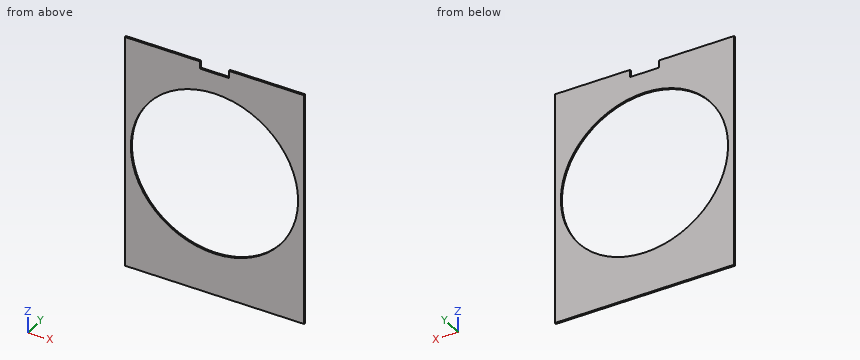
from build123d import *

# Parameters (mm, degrees)
SKETCH4_W           = 381
SKETCH4_H           = 508
BOSS_EXTRUDE1_DEPTH = 3.81
SKETCH5_R           = 177.8
CUT_EXTRUDE1_DEPTH  = 789.432041398
SKETCH6_W           = 62
SKETCH6_H           = 16
CUT_EXTRUDE2_DEPTH  = 789.432041398


with BuildPart() as part:
    # Sketch4 → Boss-Extrude1 (new body)
    with BuildSketch(Plane(origin=(190.463297595, 0, 436.273520924), x_dir=(1, 0, 0), z_dir=(0, 1, 0))):
        Rectangle(SKETCH4_W, SKETCH4_H)
    extrude(amount=BOSS_EXTRUDE1_DEPTH)

    # Sketch5 → Cut-Extrude1 (cut, through all)
    with BuildSketch(Plane(origin=(0, 3.81, 0), x_dir=(1, 0, 0), z_dir=(0, 1, 0))):
        with Locations(Location((190.463297595, -451.583397082, 0), (0, 0, 270))):
            Circle(SKETCH5_R)
    extrude(amount=-CUT_EXTRUDE1_DEPTH, mode=Mode.SUBTRACT)

    # Sketch6 → Cut-Extrude2 (cut, through all)
    with BuildSketch(Plane(origin=(0, 3.81, 0), x_dir=(1, 0, 0), z_dir=(0, 1, 0))):
        with Locations((190.463297595, -682.273520924)):
            Rectangle(SKETCH6_W, SKETCH6_H)
    extrude(amount=-CUT_EXTRUDE2_DEPTH, mode=Mode.SUBTRACT)


solid = part.part
Part model, mm, in its own coordinate system. Coordinates: 2 decimals unless noted, no trailing zeros. Loops run counter-clockwise (first coordinate to the right, second up) from the corner with the lowest first, then second, coordinate; pieces in that order, holes last. Notation, with made-up numbers: M -7.75,31.25 L 15.25,31.25 A25 cw 15.25,70.25 Z; hole C 58.25,-6 d8. An arc over 180 degrees is marked long. Use a Markdown table: item, result. Add a question column.
Q1. Cut at C-C (y = 1.85). Write the cut outline in (x, z), and give its area (3 significant figures).
Q2. Pin check, flat tip, straight feed: P1, Ø1.9, axis at x = 202.5, y = 1, coming from the +Z side. Stop position of the tip, or through.
Q3. Cut at B-B (z = 281.5). Write the cut outline in (x, y), and give its area (3 significant figures).
Q4. Probe L1, parallel to X at y = 0.55, z = 584; L2, parallel to X at y = 1.6, z = 519.5; L3, parallel to Z at x = 242, y = 2.3. List the from-to ranges inside material, lowest first.
Q5. Cut at A-A (x = 142). Write the cut outline in (y, z), and give its area (3 significant figures).
Worked out:
| question | item | result |
|---|---|---|
| 1 | outline | M -0.04,182.27 L 380.96,182.27 L 380.96,690.27 L 221.46,690.27 L 221.46,674.27 L 159.46,674.27 L 159.46,690.27 L -0.04,690.27 Z; hole C 190.46,451.58 d355.6 |
| 1 | area | 93,200 mm2 |
| 2 | P1 | stops at z = 674.27 |
| 3 | outline | M -0.04,0 L 138.65,0 L 138.65,3.81 L -0.04,3.81 Z; M 242.28,0 L 380.96,0 L 380.96,3.81 L 242.28,3.81 Z |
| 3 | area | 1,060 mm2 |
| 4 | L1 | x = -0.04 to 71.81, 309.12 to 380.96 |
| 4 | L2 | x = -0.04 to 26.15, 354.78 to 380.96 |
| 4 | L3 | z = 182.27 to 281.42, 621.75 to 690.27 |
| 5 | outline | M 0,182.27 L 3.81,182.27 L 3.81,280.52 L 0,280.52 Z; M 0,622.65 L 3.81,622.65 L 3.81,690.27 L 0,690.27 Z |
| 5 | area | 632 mm2 |
